Check sheet for the modelled part. Datum: model origin and axes. Units: mm. Round coordinates to 2 decimals unless told otherwise and drop trailing zeros. Write each loop counter-clockwise with the first axis right and the second up, starting at its lowest first coordinate (ties: lowest second). Pieces come first, ordered by that corner, then holes. Notation, with made-up numbers: M -39.5,9.25 L 10.5,9.25 A17 ccw 10.5,18.25 Z; hole C 10.25,14.25 d9. An arc over 180 degrees is marked long. One line per item, written item: value.
from build123d import *

# Parameters (mm, degrees)
SKETCH_2_R      = 2.25
SKETCH_2_R_2    = 2.368301068
EXTRUDE_2_DEPTH = 3
FILLET_2_R      = 4


with BuildPart() as part:
    # 草图2 → 凸台-拉伸2 (new body)
    with BuildSketch(Plane.XY):
        Polygon((-167.590783161, -24.567963054), (-179.98483895, 46.885925983), (-161.669401762, 62.135536129), (-105.010365497, 13.121555122), (-105.010365497, -9.480363054), (-120.053839996, -24.567963054), align=None)
        with Locations((-154.836997815, 43.253183089)):
            Circle(SKETCH_2_R, mode=Mode.SUBTRACT)
        with Locations((-164.79992885, 35.377270114)):
            Circle(SKETCH_2_R, mode=Mode.SUBTRACT)
        with Locations((-162.712910791, 53.216114124)):
            Circle(SKETCH_2_R, mode=Mode.SUBTRACT)
        with Locations((-172.675841825, 45.340201148)):
            Circle(SKETCH_2_R, mode=Mode.SUBTRACT)
        with Locations((-111.676854941, 7.182036946)):
            Circle(SKETCH_2_R, mode=Mode.SUBTRACT)
        with Locations((-124.376854941, -5.517963054)):
            Circle(SKETCH_2_R, mode=Mode.SUBTRACT)
        with Locations((-124.376854941, -19.386363054)):
            Circle(SKETCH_2_R, mode=Mode.SUBTRACT)
        with Locations((-137.076854941, -19.386363054)):
            Circle(SKETCH_2_R, mode=Mode.SUBTRACT)
        with Locations((-149.776854941, -19.386363054)):
            Circle(SKETCH_2_R, mode=Mode.SUBTRACT)
        with Locations((-162.476854941, -19.386363054)):
            Circle(SKETCH_2_R, mode=Mode.SUBTRACT)
        with Locations((-141.172189922, 5.48847701)):
            Circle(SKETCH_2_R, mode=Mode.SUBTRACT)
        with Locations((-148.489740206, 0)):
            Circle(SKETCH_2_R, mode=Mode.SUBTRACT)
        with Locations((-156.924015874, 25.414339079)):
            Circle(SKETCH_2_R, mode=Mode.SUBTRACT)
        with Locations((-164.189999825, 19.901668358)):
            Circle(SKETCH_2_R_2, mode=Mode.SUBTRACT)
        with Locations((-111.676854941, -5.517963054)):
            Circle(SKETCH_2_R, mode=Mode.SUBTRACT)
    extrude(amount=EXTRUDE_2_DEPTH)

    # 圆角2
    fillet_2_edges = [part.edges().sort_by_distance(p)[0] for p in [
        (-120.053839996, -24.567963054, 1.5),
        (-167.590783161, -24.567963054, 1.5),
        (-179.98483895, 46.885925983, 1.5),
        (-161.669401762, 62.135536129, 1.5),
        (-105.010365497, 13.121555122, 1.5),
        (-105.010365497, -9.480363054, 1.5),
    ]]
    fillet(fillet_2_edges, radius=FILLET_2_R)


solid = part.part
Q1. Sectioned sample at A-A on z = 1.9. State how many separate pieces and enclosed holes the cut face has, and give its area (3 significant figures).
Completed:
separate pieces: 1
enclosed holes: 15
area: 4,170 mm^2
Q2. Sectioned sample at C-C on x = -131. Enter the section's corners in (y, z).
Completed:
outline: M -24.57,0 L 35.6,0 L 35.6,3 L -24.57,3 Z
Q3. Draft check along X on faces 1 (the cylindrical face through (-120.2, -24.27, 1.52)), 2 (the flat face through (-173.8, 11.22, 1.48)), 3 (the cylindrical face through (-161.675, 51.22, 1.479)). Enter one of: pulls with the +X half, pulls with the -X half, needs draft (parallel to the pull), parting line crosses it, or undercut.
Completed:
face 1: pulls with the +X half
face 2: pulls with the -X half
face 3: undercut
Q4. Sectioned sample at B-B on y = 0. Enter the section's corners in (x, z), and give its area (3 significant figures).
Completed:
outline: M -171.85,0 L -150.74,0 L -150.74,3 L -171.85,3 Z; M -146.24,0 L -105.01,0 L -105.01,3 L -146.24,3 Z
area: 187 mm^2
Q5. Scan lines: line 1 (Y direction, x = -166, z = 0.9); line 2 (X direction, y = -20, z = 2.05); line 3 (Y direction, x = -150.5, z = 2.8). Record each from-to range of solid material in increasing order. Write a range as [from, to].
Completed:
line 1: [-24.15, 18.37], [21.43, 33.47], [37.28, 58.53]
line 2: [-168.38, -164.64], [-160.31, -151.94], [-147.61, -139.24], [-134.91, -126.54], [-122.21, -115.5]
line 3: [-24.57, -21.52], [-17.26, -1.01], [1.01, 52.47]
Q6. Sectioned sample at D-D on y = -9.5. Enter the section's corners in (x, z), and give its area (3 significant figures).
Completed:
outline: M -170.2,0 L -105.38,0 L -105.38,3 L -170.2,3 Z
area: 194 mm^2
Q7. Depth check by flat-ended pin: P1, Ø3.5, axis at x = -164.8, y = 35.38, coming from the +Z side. Enter the tip coordinate at first touch or a pass-through.
Completed:
P1: through
